```python
from build123d import *

# Parameters (mm, degrees)
F0_R     = 19.05
F1_DEPTH = 25.4
F3_DEPTH = 12.7
F5_DEPTH = 7.62


with BuildPart() as f1:
    # F0 (on Right) → F1 (new body)
    with BuildSketch(Plane.YZ):
        Circle(F0_R)
    extrude(amount=F1_DEPTH)

    # F2 (on face) + F0 (on Right) → F3 (cut)
    with BuildSketch(Plane.YZ.offset(25.4)):
        Polygon((13.868033, 4.767703), (2.805065, 14.39392), (-11.062968, 9.626218), (-13.868033, -4.767703), (-2.805065, -14.39392), (11.062968, -9.626218), align=None)
    with BuildSketch(Plane.YZ):
        Circle(F0_R)
    extrude(amount=-F3_DEPTH, mode=Mode.SUBTRACT)

    # F4 (on Right) → F5 (join)
    with BuildSketch(Plane.YZ):
        Polygon((3.795503, -14.165009), (14.165009, -3.795503), (10.369507, 10.369507), (-3.795503, 14.165009), (-14.165009, 3.795503), (-10.369507, -10.369507), align=None)
    extrude(amount=-F5_DEPTH)


solid = f1.part
```
Could you check a few things on this model? Use its own coordinates, in mm. A direction names the side the tool comes from. Round coordinates to 2 decimals unless told otherwise and drop trailing zeros. Loops run counter-clockwise (first coordinate to the right, second up) from the corner with the lowest first, then second, coordinate; pieces in that order, holes last.
Q1. I want a section at C-C (y = 4.5). Write out the boundary of the cut face in (x, z).
Q2. Thinking about a two-plate mould opening in Z: for faces 5 (the flat face through (-3.757, 12.294, 3.188)), 6 (the flat face through (19.139, 4.032, -12.043)), 7 (the cylindrical face through (12.52, -15.12, -11.59)), 8 (the flat face through (-7.62, 0, 0)), which applies, pulls with the +Z half, pulls with the -Z half, needs draft (parallel to the pull), parting line crosses it, or undercut?
Q3. I want a section at B-B (z = 12). Write out the boundary of the cut face in (x, y), and give its area (3 significant figures).
Q4. For P1, Ø6, axis at y = -4.5, z = -6.5, coming from the +X side; P2, Ø1, axis at x = 18.5, z = 10, coming from the +Y side; P3, Ø10, axis at x = 5, z = -3.5, coming from the +Y side; P4, Ø8, axis at x = 16, z = 5, coming from the -Y side, each with a flat end and sliding along its axis, tell me the tip position at first contact or that it passes through.
Q5. I want a section at A-A (x = 22). Write out the boundary of the cut face in (y, z), and give its area (3 significant figures).
Q6. On a 3-axis mill with a long thin cutter (end or side, diameter ignored), from which of +Z, -Z, +X, -X, +Y, -Y can I reach the whole of each face in a straight line? I mean faces 1 (the flat face through (-3.76, -3.39, -12.24)), 2 (the flat face through (19.139, 12.446, -2.53)), 3 (the flat face through (-3.76, 3.39, 12.24)), 4 (the flat face through (0, -5, -12)). Say none if no direction works.
Q7. I want a section at D-D (x = 4.5). Write out the boundary of the cut face in (y, z).
Q8. Please list where these lines run through material, in increasing order: L1, parallel to X at y = 4, z = 12.5; L2, parallel to X at y = -5, z = -1; L3, parallel to Z at x = 15.5, y = -6.
Answer below:
1. outline: (-7.62, -13.46) - (0, -13.46) - (0, -18.51) - (25.4, -18.51) - (25.4, -11.88) - (12.7, -11.88) - (12.7, 12.92) - (25.4, 12.92) - (25.4, 18.51) - (0, 18.51) - (0, 11.94) - (-7.62, 11.94) - close
2. face 5: pulls with the +Z half
2. face 6: undercut
2. face 7: parting line crosses it
2. face 8: needs draft
3. outline: (-7.62, -5.96) - (0, -5.96) - (0, -14.8) - (25.4, -14.8) - (25.4, -4.16) - (12.7, -4.16) - (12.7, 5.56) - (25.4, 5.56) - (25.4, 14.8) - (0, 14.8) - (0, 4.28) - (-7.62, 4.28) - close
3. area: 706 mm2
4. P1: stops at x = 12.7
4. P2: stops at y = 16.51
4. P3: stops at y = 19.05
4. P4: stops at y = -19.02
5. outline: circle Ø38.1 at (0, 0); hole (-13.87, -4.77) - (-2.81, -14.39) - (11.06, -9.63) - (13.87, 4.77) - (2.81, 14.39) - (-11.06, 9.63) - close
5. area: 581 mm2
6. face 1: -Z, -X, -Y
6. face 2: +X
6. face 3: +Z, -X, +Y
6. face 4: -X
7. outline: circle Ø38.1 at (0, 0)
8. L1: x = 0 to 12.7
8. L2: x = -7.62 to 12.7
8. L3: z = -18.08 to -11.61, 11.37 to 18.08
